Could you check a few things on this model? Use its own coordinates, in mm. A direction names the side the tool comes from. Coordinates: 2 decimals unless noted, no trailing zeros. Write each loop counter-clockwise with the first axis right and the second up, starting at its lowest first coordinate (ties: lowest second). Pieces come first, ordered by that corner, then holes.
```python
from build123d import *

# Parameters (mm, degrees)
SKETCH2_W           = 60
SKETCH2_H           = 100
SKETCH2_R           = 1.5
SKETCH2_W_2         = 3.5
SKETCH2_H_2         = 85
SKETCH2_W_3         = 35
SKETCH2_H_3         = 3.5
BOSS_EXTRUDE1_DEPTH = 3
FILLET1_R           = 2


with BuildPart() as part:
    # Sketch2 → Boss-Extrude1 (new body)
    with BuildSketch(Plane.XY):
        with Locations((0.630630631, -28.711797537)):
            Rectangle(SKETCH2_W, SKETCH2_H)
        with Locations((-24.369369369, -74.961797537)):
            Circle(SKETCH2_R, mode=Mode.SUBTRACT)
        with Locations((-24.369369369, -28.711797537)):
            Circle(SKETCH2_R, mode=Mode.SUBTRACT)
        with Locations((-15.619369369, -28.711797537)):
            Rectangle(SKETCH2_W_2, SKETCH2_H_2, mode=Mode.SUBTRACT)
        with Locations((5.630630631, -74.961797537)):
            Rectangle(SKETCH2_W_3, SKETCH2_H_3, mode=Mode.SUBTRACT)
        with Locations((26.880630631, -28.711797537)):
            Rectangle(SKETCH2_W_2, SKETCH2_H_2, mode=Mode.SUBTRACT)
        with Locations((-24.369369369, 17.538202463)):
            Circle(SKETCH2_R, mode=Mode.SUBTRACT)
        with Locations((5.630630631, -28.711797537)):
            Rectangle(SKETCH2_W_3, SKETCH2_H_2, mode=Mode.SUBTRACT)
        with Locations((5.630630631, 17.538202463)):
            Rectangle(SKETCH2_W_3, SKETCH2_H_3, mode=Mode.SUBTRACT)
    extrude(amount=BOSS_EXTRUDE1_DEPTH)

    # Fillet1
    # the kernel refuses this fillet: 2 mm, written as the material it adds along each edge
    with BuildSketch(Plane(origin=(-11.869369369, 15.788202463, 0), x_dir=(1, 0, 0), z_dir=(0, 0, 1)), Plane(origin=(23.130630631, 19.288202463, 0), x_dir=(-1, 0, 0), z_dir=(0, 0, 1)), Plane(origin=(-11.869369369, 19.288202463, 0), x_dir=(0, -1, 0), z_dir=(0, 0, 1)), Plane(origin=(-17.369369369, 13.788202463, 0), x_dir=(0, -1, 0), z_dir=(0, 0, 1)), Plane(origin=(25.130630631, 13.788202463, 0), x_dir=(0, -1, 0), z_dir=(0, 0, 1)), Plane(origin=(28.630630631, 13.788202463, 0), x_dir=(-1, 0, 0), z_dir=(0, 0, 1)), Plane(origin=(-13.869369369, 13.788202463, 0), x_dir=(-1, 0, 0), z_dir=(0, 0, 1)), Plane(origin=(-13.869369369, -71.211797537, 0), x_dir=(0, 1, 0), z_dir=(0, 0, 1)), Plane(origin=(25.130630631, -71.211797537, 0), x_dir=(1, 0, 0), z_dir=(0, 0, 1)), Plane(origin=(-11.869369369, -76.711797537, 0), x_dir=(1, 0, 0), z_dir=(0, 0, 1)), Plane(origin=(23.130630631, -73.211797537, 0), x_dir=(-1, 0, 0), z_dir=(0, 0, 1)), Plane(origin=(23.130630631, -76.711797537, 0), x_dir=(0, 1, 0), z_dir=(0, 0, 1))) as fillet1_piece_1:
        with BuildLine():
            CenterArc((FILLET1_R, FILLET1_R), FILLET1_R, 180, 90)
            Line((0, FILLET1_R), (0, 0))
            Line((0, 0), (FILLET1_R, 0))
        make_face()
    extrude(amount=3)
    with BuildSketch(Plane(origin=(23.130630631, 15.788202463, 0), x_dir=(-1, 0, 0), z_dir=(0, 0, 1)), Plane(origin=(28.630630631, -71.211797537, 0), x_dir=(-1, 0, 0), z_dir=(0, 0, 1)), Plane(origin=(-17.369369369, -71.211797537, 0), x_dir=(0, 1, 0), z_dir=(0, 0, 1)), Plane(origin=(-11.869369369, -73.211797537, 0), x_dir=(1, 0, 0), z_dir=(0, 0, 1))) as fillet1_piece_2:
        with BuildLine():
            CenterArc((FILLET1_R, -FILLET1_R), FILLET1_R, 90, 90)
            Line((0, -FILLET1_R), (0, 0))
            Line((0, 0), (FILLET1_R, 0))
        make_face()
    extrude(amount=3)


solid = part.part
```
Item 1: If I drill on line 1 along X through (y, z) = (4, 2.8); line 2 along Y through (x, z) = (12, 0.2); line 3 along X through (y, z) = (-27.5, 2.25), over which ranges is the centre line in solid material (lowest first)?
Item 2: Which directions (+Z, -Z, +X, -X, +Y, -Y) give clear straight access to the entire face, cutting with the end or side of a thin tool? Please do faces 1 (the flat face through (-13, -18, 3)), 2 (the cylindrical face through (-16.9, -70.5, 1.5)).
Item 3: I want a section at A-A, the plane y = -62. List the corners of the cut face in (x, z) for me.
Item 4: I want a section at B-B, the plane x = 3. List the corners of the cut face in (y, z) for me.
Item 5: If we mould it in two halves opening along Y, with no side actions, what happens to faces 3 (the flat face through (5, 15.788, 1)), 4 (the flat face through (-29.369, -29, 1)), 5 (the flat face through (0, -78.712, 1))? For each: released by +Y, released by -Y, zero draft, split by the parting line, or undercut.
Item 6: I want a section at C-C, the plane z = 2.4. Count the separate pieces of the cut face and the enclosed holes in it, then the cut area to 3 significant figures.
Taken from the geometry:
1. line 1: x = -29.37 to -17.37, -13.87 to -11.87, 23.13 to 25.13, 28.63 to 30.63
1. line 2: y = -78.71 to -76.71, -73.21 to -71.21, 13.79 to 15.79, 19.29 to 21.29
1. line 3: x = -29.37 to -25.25, -23.49 to -17.37, -13.87 to -11.87, 23.13 to 25.13, 28.63 to 30.63
2. face 1: +Z, +X, -X, +Y, -Y
2. face 2: +Z, -Z
3. outline: (-29.37, 0) - (-17.37, 0) - (-17.37, 3) - (-29.37, 3) - close; (-13.87, 0) - (-11.87, 0) - (-11.87, 3) - (-13.87, 3) - close; (23.13, 0) - (25.13, 0) - (25.13, 3) - (23.13, 3) - close; (28.63, 0) - (30.63, 0) - (30.63, 3) - (28.63, 3) - close
4. outline: (-78.71, 0) - (-76.71, 0) - (-76.71, 3) - (-78.71, 3) - close; (-73.21, 0) - (-71.21, 0) - (-71.21, 3) - (-73.21, 3) - close; (13.79, 0) - (15.79, 0) - (15.79, 3) - (13.79, 3) - close; (19.29, 0) - (21.29, 0) - (21.29, 3) - (19.29, 3) - close
5. face 3: undercut
5. face 4: zero draft
5. face 5: released by -Y
6. separate pieces: 1
6. enclosed holes: 8
6. area: 2,180 mm2
